from build123d import *

# Parameters (mm, degrees)
F1_DEPTH = 5
F2_T     = -3
F3_SIZE  = 2
F4_W     = 5.3098537028
F4_H     = 10
F5_DEPTH = 1.5


# Not quite as in the source:
# - a pattern or mirror of a feature is missing from the dataset's text; its kind, count and spacing are read off the source's solid


with BuildPart() as f1:
    # F0 (on Top) → F1 (new body, symmetric)
    with BuildSketch(Plane.XY):
        Polygon((53.696885705, 32.7549055219), (0, 32.7549055219), (-53.696885705, 32.7549055219), (-53.696885705, 0), (-53.696885705, -32.7549055219), (0, -32.7549055219), (53.696885705, -32.7549055219), (53.696885705, 0), align=None)
    extrude(amount=F1_DEPTH, both=True)

    # F2
    f2_openings = [f1.faces().sort_by_distance(p)[0] for p in [
        (0, 0, 5),
    ]]
    offset(amount=F2_T, openings=f2_openings)

    # F3
    f3_edges = [f1.edges().sort_by_distance(p)[0] for p in [
        (53.696886, -32.754906, 0),
        (-53.696886, 32.754906, 0),
        (53.696886, 32.754906, 0),
        (-53.696886, -32.754906, 0),
    ]]
    chamfer(f3_edges, length=F3_SIZE)

    # F4 (on face) → F5 (join)
    with BuildSketch(Plane.XZ.offset(32.7549055219)):
        with Locations((-42.1222578734, 0)):
            Rectangle(F4_W, F4_H)
        with Locations((-31.5025504678, 0)):
            Rectangle(F4_W, F4_H)
        with Locations((-20.8828430623, 0)):
            Rectangle(F4_W, F4_H)
    f5 = extrude(amount=F5_DEPTH)

    # F5_copies: F5 across plane
    add(f5.mirror(Plane(origin=(0, 0, 0), x_dir=(0, 0, 1), z_dir=(1, 0, 0))))


solid = f1.part
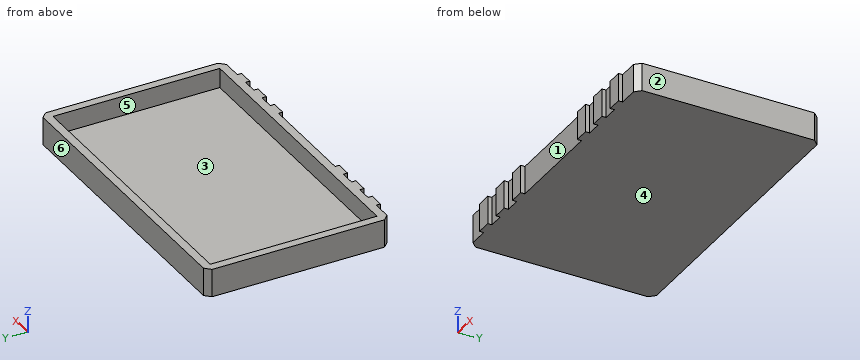
Can you work these out from the model? Positions are in its coordinate system, mm. Face numbers are marked on the shaded views. A direction names the side the tool comes from. Coordinates: 2 decimals unless noted, no trailing zeros. Write each loop counter-clockwise with the first axis right and the second up, starting at its lowest first coordinate (ties: lowest second). Pieces come first, ordered by that corner, then holes. Notation, with made-up numbers: (60, 14) -> (70, 14) arc R20 cw to (70, 21) -> close; hole circle Ø6 at (44.25, -23). An arc over 180 degrees is marked (long way). Answer as CSV lines item,"result".
1) If we section it at B-B on y = 3: Please give me the cut outline in (x, z).
Check result:
outline,"(-53.7, -5) -> (53.7, -5) -> (53.7, 5) -> (50.7, 5) -> (50.7, -2) -> (-50.7, -2) -> (-50.7, 5) -> (-53.7, 5) -> close"
2) If I drill on line 1 (Y direction, x = -39, z = 4); line 2 (Y direction, x = -39.5, z = 2); line 3 (X direction, y = -29, z = 3.75), over which ranges is the centre line in solid material (lowest first)? Write a range as from..to.
Check result:
line 1,"-32.75..-29.75, 29.75..32.75"
line 2,"-34.25..-29.75, 29.75..32.75"
line 3,"-53.7..-50.7, 50.7..53.7"
3) On a 3-axis mill with a long thin cutter (end or side, diameter ignored), from which of +Z, -Z, +X, -X, +Y, -Y can I reach the whole of each face in a straight line? I mean the marked faces 1 and 2. Say none if no direction works.
Check result:
face 1,"+Z, -Z, -Y"
face 2,"+Z, -Z, +X, +Y, -Y"
4) Will these pins go through, and if not, where does the flat tip stop? P1, Ø1.6, axis at y = -33.5, z = -0.5, coming from the -X side; P2, Ø3, axis at x = -39, z = 2.5, coming from the -Y side; P3, Ø5.5, axis at x = -48.5, z = 1, coming from the -Y side; P4, Ø1.2, axis at y = -34, z = -1, coming from the +X side.
Check result:
P1,"x = -51.75"
P2,"y = -34.25"
P3,"y = -32.75"
P4,"x = 44.78"
5) If we mould it in two halves opening along Y, with no side actions, what happens to the marked faces 3, 4, 5 and 6? For each: +Y half, -Y half, draft (parallel to the pull), parting line (faces both ways), or undercut.
Check result:
face 3,"undercut"
face 4,"draft"
face 5,"undercut"
face 6,"+Y half"
6) If we section it at A-A on x = 13: Please give me the cut outline in (y, z), then the cut area to 3 significant figures.
Check result:
outline,"(-32.75, -5) -> (32.75, -5) -> (32.75, 5) -> (29.75, 5) -> (29.75, -2) -> (-29.75, -2) -> (-29.75, 5) -> (-32.75, 5) -> close"
area,"239 mm²"
